Drawing for the job (mm, zero at the part's lowest x, y, z). A direction names the side the tool comes from. Round coordinates to 2 decimals unless told otherwise and drop trailing zeros. Loops run counter-clockwise (first coordinate to the right, second up) from the corner with the lowest first, then second, coordinate; pieces in that order, holes last. Notation, with made-up numbers: (-29, 36.5) - (-15, 36.5) arc R24 ccw to (-15, 55.5) - close; hole circle Ø6 at (79.5, 48). An arc over 180 degrees is marked (long way). Put each result on its own line as item: value.
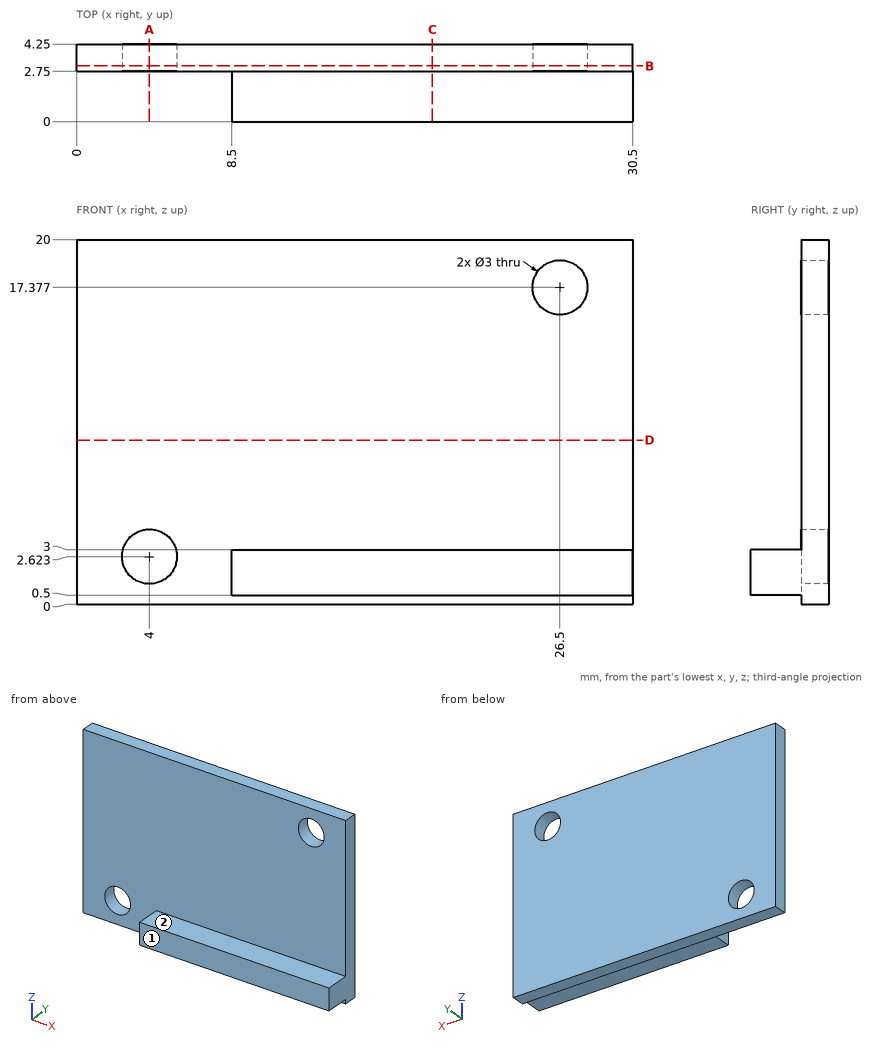
1. Band-saw the part on C-C (x = 19.5). List the corners of the cut face in (y, z).
A:
outline: (0, 0.5) - (2.75, 0.5) - (2.75, 0) - (4.25, 0) - (4.25, 20) - (2.75, 20) - (2.75, 3) - (0, 3) - close
2. Probe line 1 along Y through (x, z) = (19, 13); line 2 along X through (y, z) = (0.9, 1); line 3 along Z through (x, y) = (11, 2.2). List the from-to ranges inside material, lowest first. Write a range as [from, to].
A:
line 1: y = [2.75, 4.25]
line 2: x = [8.5, 30.5]
line 3: z = [0.5, 3]
3. Band-saw the part on B-B (y = 3.05). List the corners of the cut face in (x, z), plus the area to 3 significant figures.
A:
outline: (0, 0) - (30.5, 0) - (30.5, 20) - (0, 20) - close; hole circle Ø3 at (4, 2.62); hole circle Ø3 at (26.5, 17.38)
area: 596 mm²
4. Band-saw the part on A-A (x = 4). List the corners of the cut face in (y, z).
A:
outline: (2.75, 0) - (4.25, 0) - (4.25, 1.12) - (2.75, 1.12) - close; (2.75, 4.12) - (4.25, 4.12) - (4.25, 20) - (2.75, 20) - close
5. Tool access for the marked faces 1 and 2: list every direction of +Z, -Z, +X, -X, +Y, -Y with a clear straight run to the whole face (end or side of a thin tool).
A:
face 1: +Z, -Z, +X, -X, -Y
face 2: +Z, +X, -X, -Y
6. Band-saw the part on D-D (z = 9). List the corners of the cut face in (x, y).
A:
outline: (0, 2.75) - (30.5, 2.75) - (30.5, 4.25) - (0, 4.25) - close
7. Pin check, flat tips, straight feed: P1, Ø2.5, axis at x = 4, z = 2.62, coming from the -Y side; P2, Ø5, axis at x = 5.5, z = 9, coming from the -Y side; P3, Ø0.8, axis at x = 16, y = 1.5, coming from the +Z side; P4, Ø1.4, axis at x = 21.5, y = 2, coming from the -Z side. Stop position of each tip, or through.
A:
P1: passes through
P2: stops at y = 2.75
P3: stops at z = 3
P4: stops at z = 0.5
